The listing builds one solid part. Answer for the finished solid, in the listing's coordinates (mm). A direction names the side the tool comes from. Round coordinates to 2 decimals unless told otherwise and drop trailing zeros. Order: outer loops, then holes, each group sorted by start corner. A loop starts at its lowest first (then second) coordinate and runs counter-clockwise, first axis right, second up. Notation, with made-up numbers: (33, -8.5) - (82, -8.5) arc R30 ccw to (82, 18.5) - close; hole circle Ø1 at (-19, 67.25). An arc over 180 degrees is marked (long way). Use CSV: the item, a comma, the result in double quotes. Start each with the question number.
Item 1: Find section B-B, the plane y = -11. Give the vertices of the cut face in (x, z).
Item 2: Find section D-D, the plane z = 19. Give the vertices of the cut face in (x, y), plus the area to 3 significant figures.
Item 3: Flat-ended cylindrical pins translate along their axes: P1, Ø17.5, axis at x = 3, z = 36.5, coming from the -Y side; P2, Ø9.5, axis at x = 0, y = 0, coming from the -Z side; P3, Ø6.5, axis at y = -4, z = 15.5, coming from the -X side; P4, Ø3, axis at x = 0, z = 9, coming from the +Y side. Find the tip coordinate at first contact, or state that the pin passes through.
Item 4: Find section C-C, the plane x = 0. Give the vertices of the cut face in (y, z).
Item 5: For faces 4 (the cylindrical face through (-0.224, -6.796, 49.782)), 5 (the cylindrical face through (-14.643, -8.986, 7.809)), 6 (the conical face through (0.227, -6.87, 9.174)), 7 (the flat face through (-6, -7, 8)), 8 (the flat face through (14, -8, 8)), determine the directions among +Z, -Z, +X, -X, +Y, -Y from which every point of the face is accessible in a straight line to the end or side of a thin tool.
Item 6: Find section A-A, the plane x = 17.5. Give the vertices of the cut face in (y, z), plus the area to 3 significant figures.
Item 7: Determine the mould class of faces 1 (the flat face through (0, -8, 0)), 2 (the flat face through (16, -10, 8)), 3 (the cylindrical face through (0.221, -6.696, 4.437)) for opening direction Z: +Z half, -Z half, draft (parallel to the pull), parting line (faces both ways), or undercut.
Item 8: Straight lines are drawn through the part: line 1 along X through (y, z) = (6, 11.5); line 2 along Z through (x, y) = (-17.5, -9.25); line 3 along Z through (x, y) = (-17.5, -12.55). For each, find the intervals that lie inside material, in ascending order. Write a range as [from, to].
```python
from build123d import *

# Parameters (mm, degrees)
CYLINDER003_R     = 1.5
CYLINDER003_DEPTH = 8
CYLINDER002_R     = 8
CYLINDER002_DEPTH = 3
CYLINDER001_R     = 8
CYLINDER001_DEPTH = 3
CYLINDER_R        = 8
CYLINDER_DEPTH    = 5
PAD_DEPTH         = 52
SKETCH005_R       = 6.8
POCKET_DEPTH      = 25
SKETCH006_R       = 6.7
POCKET001_DEPTH   = 25
PAD002_DEPTH      = 32
SKETCH010_R       = 1.5
POCKET004_DEPTH   = 8
PAD001_DEPTH      = 20
SKETCH008_R       = 2.1
POCKET002_DEPTH   = 7
SKETCH009_R       = 3.6
POCKET003_DEPTH   = 2
FILLET_R          = 5
FILLET001_R       = 2.1
CHAMFER_SIZE      = 1


with BuildPart() as zylinder003:
    # Cylinder003 → Cylinder003 (new body)
    with BuildSketch(Plane(origin=(-6, -7.5, 0), x_dir=(1, 0, 0), z_dir=(0, 0, 1))):
        Circle(CYLINDER003_R)
    extrude(amount=CYLINDER003_DEPTH)


with BuildPart() as zylinder002:
    # Cylinder002 → Cylinder002 (new body)
    with BuildSketch(Plane.XY.offset(43.5)):
        Circle(CYLINDER002_R)
    extrude(amount=CYLINDER002_DEPTH)


with BuildPart() as zylinder001:
    # Cylinder001 → Cylinder001 (new body)
    with BuildSketch(Plane.XY.offset(33.5)):
        Circle(CYLINDER001_R)
    extrude(amount=CYLINDER001_DEPTH)


with BuildPart() as zylinder:
    # Cylinder → Cylinder (new body)
    with BuildSketch(Plane.XY.offset(10)):
        Circle(CYLINDER_R)
    extrude(amount=CYLINDER_DEPTH)


with BuildPart() as pocket004:
    # Sketch → Pad (new body)
    with BuildSketch(Plane.XY):
        with BuildLine():
            ThreePointArc((-7.071068, 7.071068), (0, -10), (7.071068, 7.071068))
            Line((7.071068, 7.071068), (4.242641, 4.242641))
            ThreePointArc((-4.242641, 4.242641), (0, -6), (4.242641, 4.242641))
            Line((-4.242641, 4.242641), (-7.071068, 7.071068))
        make_face()
    extrude(amount=PAD_DEPTH)

    # Sketch005 → Pocket (cut)
    with BuildSketch(Plane.XY.offset(52)):
        Circle(SKETCH005_R)
    extrude(amount=-POCKET_DEPTH, mode=Mode.SUBTRACT)

    # Sketch006 → Pocket001 (cut)
    with BuildSketch(Plane(origin=(0, 0, 0), x_dir=(1, 0, 0), z_dir=(0, 0, -1))):
        Circle(SKETCH006_R)
    extrude(amount=-POCKET001_DEPTH, mode=Mode.SUBTRACT)

    # Sketch007 → Pad002 (new body)
    with BuildSketch(Plane.XY.offset(52)):
        with BuildLine():
            ThreePointArc((-10, 0), (0, -10), (10, 0))
            Line((10, 0), (10, -10.1))
            Line((-10, -10.1), (10, -10.1))
            Line((-10, 0), (-10, -10.1))
        make_face()
    extrude(amount=-PAD002_DEPTH)

    # Cut: cut Zylinder
    add(zylinder.part, mode=Mode.SUBTRACT)

    # Cut001: cut Zylinder001
    add(zylinder001.part, mode=Mode.SUBTRACT)

    # Cut002: cut Zylinder002
    add(zylinder002.part, mode=Mode.SUBTRACT)

    # Sketch010 → Pocket004 (cut)
    with BuildSketch(Plane.XY.offset(52)):
        with Locations((-6, -7.493998)):
            Circle(SKETCH010_R)
    extrude(amount=-POCKET004_DEPTH, mode=Mode.SUBTRACT)


with BuildPart() as chamfer_body:
    # Sketch003 → Pad001 (new body)
    with BuildSketch(Plane.XY):
        with BuildLine():
            ThreePointArc((-10, 0), (0, -10), (10, 0))
            Line((10, 0), (10, -8))
            Line((10, -8), (25, -8))
            Line((25, -8), (25, -15))
            Line((-25, -15), (25, -15))
            Line((-25, -8), (-25, -15))
            Line((-10, -8), (-25, -8))
            Line((-10, 0), (-10, -8))
        make_face()
    extrude(amount=PAD001_DEPTH)

    # Sketch008 → Pocket002 (cut)
    with BuildSketch(Plane.XZ.offset(15)):
        with Locations((-17.5, 10)):
            Circle(SKETCH008_R)
        with Locations((17.5, 10)):
            Circle(SKETCH008_R)
    extrude(amount=-POCKET002_DEPTH, mode=Mode.SUBTRACT)

    # Sketch009 → Pocket003 (cut)
    with BuildSketch(Plane(origin=(0, -8, 0), x_dir=(-1, 0, 0), z_dir=(0, 1, 0))):
        with Locations((-17.5, 10)):
            Circle(SKETCH009_R)
        with Locations((17.5, 10)):
            Circle(SKETCH009_R)
    extrude(amount=-POCKET003_DEPTH, mode=Mode.SUBTRACT)

    # Fusion: union Pocket004
    add(pocket004.part)

    # Cut003: cut Zylinder003
    add(zylinder003.part, mode=Mode.SUBTRACT)

    # Fillet
    fillet_edges = [chamfer_body.edges().sort_by_distance(p)[0] for p in [
        (-25, -11.5, 20),
        (25, -11.5, 20),
    ]]
    fillet(fillet_edges, radius=FILLET_R)

    # Fillet001
    fillet001_edges = [chamfer_body.edges().sort_by_distance(p)[0] for p in [
        (10, -10.1, 36),
        (-10, -10.1, 36),
    ]]
    fillet(fillet001_edges, radius=FILLET001_R)

    # Chamfer
    chamfer_edges = [chamfer_body.edges().sort_by_distance(p)[0] for p in [
        (-2.563979, -6.189993, 15),
        (-2.563979, -6.189993, 10),
        (-2.602247, -6.282381, 33.5),
        (-2.602247, -6.282381, 36.5),
        (-2.602247, -6.282381, 43.5),
        (-2.602247, -6.282381, 46.5),
    ]]
    chamfer(chamfer_edges, length=CHAMFER_SIZE)


solid = chamfer_body.part
```
Worked out:
1,outline,"(-25, 0) - (25, 0) - (25, 15) arc R5 ccw to (20, 20) - (-20, 20) arc R5 ccw to (-25, 15) - close; hole circle Ø4.2 at (-17.5, 10); hole circle Ø4.2 at (17.5, 10)"
2,outline,"(-23, -15) - (23, -15) - (23, -8) - (10, -8) - (10, 0) arc R10 ccw to (7.07, 7.07) - (4.74, 4.74) arc R6.7 cw (long way) to (-4.74, 4.74) - (-7.07, 7.07) arc R10 ccw to (-10, 0) - (-10, -8) - (-23, -8) - close"
2,area,"455 mm²"
3,P1,"stops at y = -10.1"
3,P2,"passes through"
3,P3,"stops at x = -10"
3,P4,"stops at y = -6.53"
4,outline,"(-15, 0) - (-6.7, 0) - (-6.7, 9) - (-7.7, 10) - (-8, 10) - (-8, 15) - (-7.7, 15) - (-6.7, 16) - (-6.7, 25) - (-6, 25) - (-6, 27) - (-6.8, 27) - (-6.8, 32.5) - (-7.8, 33.5) - (-8, 33.5) - (-8, 36.5) - (-7.8, 36.5) - (-6.8, 37.5) - (-6.8, 42.5) - (-7.8, 43.5) - (-8, 43.5) - (-8, 46.5) - (-7.8, 46.5) - (-6.8, 47.5) - (-6.8, 52) - (-10.1, 52) - (-10.1, 20) - (-15, 20) - close"
5,face 4,"+Z"
5,face 5,"+Y"
5,face 6,"none"
5,face 7,"-Z"
5,face 8,"+Z, -Z, +X, +Y"
6,outline,"(-15, 0) - (-8, 0) - (-8, 6.4) - (-10, 6.4) - (-10, 7.9) - (-15, 7.9) - close; (-15, 12.1) - (-10, 12.1) - (-10, 13.6) - (-8, 13.6) - (-8, 20) - (-15, 20) - close"
6,area,"105 mm²"
7,face 1,"-Z half"
7,face 2,"undercut"
7,face 3,"draft"
8,line 1,"x = [-8, -6], [6, 8]"
8,line 2,"z = [0, 6.4], [13.6, 20]"
8,line 3,"z = [0, 7.9], [12.1, 20]"
